Autodesk Inventor part; units mm, degrees
ref_plane "YZ Plane" through (0, 0, 0) normal (1, 0, 0) x (0, 1, 0)
ref_plane "XZ Plane" through (0, 0, 0) normal (0, 1, 0) x (-1, 0, 0)
ref_plane "XY Plane" through (0, 0, 0) normal (0, 0, 1) x (1, 0, 0)
sketch "スケッチ1" plane through (0, 0, 0) normal (0, 0, 1) x (1, 0, 0)
  line L0 (-19.75, 25.75) -> (19.75, 25.75) construction
  line L1 (19.75, 25.75) -> (19.75, -25.75) construction
  line L2 (19.75, -25.75) -> (-19.75, -25.75) construction
  line L3 (-19.75, -25.75) -> (-19.75, 25.75) construction
  line L4 (-19.75, 25.75) -> (19.75, -25.75) construction
  line L5 (19.75, 25.75) -> (-19.75, -25.75) construction
  circle A0 centre (24.75, -24.25) radius 2.05
  circle A1 centre (-7.25, -4.25) radius 3.275
  line L6 (0, 25.75) -> (0, -25.75) construction
  line L7 (-19.75, 3.25) -> (-22.75, 3.25)
  line L8 (-22.75, 3.25) -> (-22.75, -4.75)
  arc A2 (-19.75, 3.25) -> (-19.75, 5.35) centre (-19.75, 4.3) ccw
  line L9 (-22.75, -0.75) -> (-19.75, -0.75) construction
  line L10 (-19.75, -4.75) -> (-22.75, -4.75)
  arc A3 (-19.75, -6.85) -> (-19.75, -4.75) centre (-19.75, -5.8) ccw
  line L11 (-19.75, 5.35) -> (-19.75, 9.25)
  line L12 (-19.75, 9.25) -> (19.75, 9.25)
  arc A4 (19.75, 5.35) -> (19.75, 3.25) centre (19.75, 4.3) ccw
  arc A5 (19.75, -4.75) -> (19.75, -6.85) centre (19.75, -5.8) ccw
  line L13 (19.75, 5.35) -> (19.75, 9.25)
  arc A6 (22.2819, -29.7189) -> (27.2181, -18.7811) centre (24.75, -24.25) ccw
  line L14 (-19.75, -6.85) -> (-19.75, -10.75)
  line L15 (-19.75, -10.75) -> (22.2819, -29.7189)
  line L16 (19.75, -6.85) -> (19.75, -15.4108)
  line L17 (19.75, -15.4108) -> (27.2181, -18.7811)
  circle A7 centre (-7.25, -4.25) radius 6 construction
  circle A8 centre (24.75, -24.25) radius 6 construction
  line L18 (2.75, 5.25) -> (14.75, 5.25)
  line L19 (14.75, 5.25) -> (14.75, -13.1543)
  line L20 (14.75, -13.1543) -> (2.75, -7.7388)
  line L21 (2.75, -7.7388) -> (2.75, 5.25)
  line L22 (19.75, 3.25) -> (22.75, 3.25)
  line L23 (22.75, 3.25) -> (22.75, -4.75)
  line L24 (22.75, -4.75) -> (19.75, -4.75)
  point P0 (0, 0)
  dimension "d0" = 39.5
  dimension "d1" = 51.5
  dimension "d2" = 4.1
  dimension "d3" = 6.55
  dimension "d4" = 32
  dimension "d5" = 20
  dimension "d6" = 3
  dimension "d7" = 1.05
  dimension "d8" = 8
  dimension "d9" = 26.5
  dimension "d11" = 30
  dimension "d12" = 12.5
  dimension "d13" = 6
  dimension "d14" = 12
  dimension "d19" = 12
  dimension "d21" = 4
  dimension "d22" = 5
  dimension "d24" = 4
  dimension "d26" = 3
extrude "押し出し1" add sketch "スケッチ1" along normal blind 2
fillet "フィレット1" radius 3.5 1 edges at (19.75, -15.4108, 1)
fillet "フィレット2" radius 1 4 edges at (2.75, 5.25, 1) (14.75, 5.25, 1) (2.75, -7.7388, 1) (14.75, -13.1543, 1)
equation "\"d24\" = d21"
properties part number "Leg_joint_pitch_frame" material "アルミニウム 2014-T4"
Input: part model. Units: mm. Frame: model coordinates. A direction names the side the tool comes from. Round coordinates to 2 decimals unless told otherwise and drop trailing zeros. Loops run counter-clockwise (first coordinate to the right, second up) from the corner with the lowest first, then second, coordinate; pieces in that order, holes last. Notation, with made-up numbers: (-36.75, 5) -> (4.25, 5) arc R16 ccw to (4.25, 18) -> close; hole circle Ø2 at (49.25, 47). An arc over 180 degrees is marked (long way). Use one line per item in the form item = value. Start each with the question number.
Item 1: Section query A-A on y = 1. Return the cut outline in (x, z).
Item 2: Contact query for flat-ended pins moving along their axis: pin 1 Ø1 at (y, z) = (7, 0.5) entering from -X; pin 2 Ø0.6 at (y, z) = (6.5, 0.5) entering from +X; pin 3 Ø0.6 at (x, z) = (10.5, 1) entering from -Y. Output: stop coordinate, or through.
Item 3: Section query B-B on z = 1.65. Count the separate pieces of the cut face and the enclosed holes in it, then the cut area to 3 significant figures.
Item 4: Mould query, pull axis X, two halves, no side actions, for faces 1 (the face through (14.281, -12.453, 1.014)), 2 (the face through (-10.522, -4.394, 0.986)), 3 (the face through (-19.75, 7, 1)), 4 (the face through (-21, -4.75, 1)). Classes: pulls with the +X half, pulls with the -X half, needs draft (parallel to the pull), parting line crosses it, or undercut.
Item 5: Set-up query: faces 5 (the face through (21, 3.25, 1)), 6 (the face through (0, 9.25, 1)), 7 (the face through (24.476, -17.544, 0.986)), 8 (the face through (4, -10, 0)), 9 (the face through (2.75, -2, 1)). Return all of +Z, -Z, +X, -X, +Y, -Y with unobstructed straight access to the full face (end or side cutting, diameter ignored); none if empty.
Item 6: Section query C-C on x = 24.75. Return the cut outline in (y, z), then the cut area to 3 significant figures.
Item 7: Section query D-D on y = 6. Return the cut outline in (x, z).
Item 8: Material intervals for L1, parallel to X at y = 1.5, z = 0.15; L2, parallel to X at y = -4, z = 0.2; L3, parallel to Y at x = 22, z = 1.7, sorted ascending. Write a range as from..to.
Ans:
q1.outline = (-22.75, 0) -> (2.75, 0) -> (2.75, 2) -> (-22.75, 2) -> close; (14.75, 0) -> (22.75, 0) -> (22.75, 2) -> (14.75, 2) -> close
q2.pin_1 = -19.75
q2.pin_2 = 19.75
q2.pin_3 = -24.54
q3.separate_pieces = 1
q3.enclosed_holes = 3
q3.area = 1,070 mm^2
q4.face_1 = undercut
q4.face_2 = undercut
q4.face_3 = pulls with the -X half
q4.face_4 = needs draft
q5.face_5 = +Z, -Z, +X, +Y
q5.face_6 = +Z, -Z, +X, -X, +Y
q5.face_7 = +Z, -Z, +X
q5.face_8 = -Z, +X, -X, +Y, -Y
q5.face_9 = +Z, -Z
q6.outline = (-30.25, 0) -> (-26.3, 0) -> (-26.3, 2) -> (-30.25, 2) -> close; (-22.2, 0) -> (-17.67, 0) -> (-17.67, 2) -> (-22.2, 2) -> close
q6.area = 17.0 mm^2
q7.outline = (-19.75, 0) -> (19.75, 0) -> (19.75, 2) -> (-19.75, 2) -> close
q8.L1 = -22.75..2.75, 14.75..22.75
q8.L2 = -22.75..-10.52, -3.98..2.75, 14.75..22.75
q8.L3 = -29.59..-16.43, -4.75..3.25
